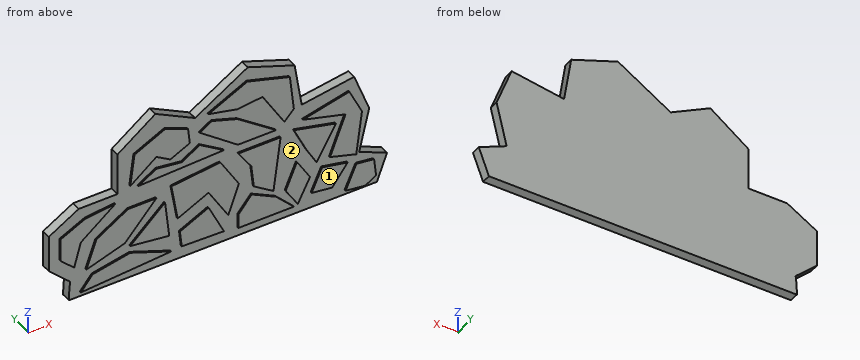
from build123d import *

# Parameters (mm, degrees)
F1_DEPTH = 3
F3_DEPTH = 0.5


with BuildPart() as f1:
    # F0 (on Front) → F1 (new body)
    with BuildSketch(Plane.XZ):
        with BuildLine():
            ThreePointArc((-49.601689, 6.298609), (-49.900323, 3.155595), (-50, 0))
            Line((-50, 0), (50, 0))
            Line((50, 0), (53.269234, 8.75))
            Line((53.269234, 8.75), (44.23077, 12.788462))
            Line((44.23077, 12.788462), (47.500003, 26.634617))
            Line((47.500003, 26.634617), (42.601875, 39.515073))
            Line((42.601875, 39.515073), (25.576925, 36.826923))
            Line((25.576925, 36.826923), (23.269232, 51.44231))
            Line((23.269232, 51.44231), (8.076922, 57.019234))
            Line((8.076922, 57.019234), (-9.038462, 46.442311))
            Line((-9.038462, 46.442311), (-21.923078, 53.17308))
            Line((-21.923078, 53.17308), (-34.230769, 44.134621))
            Line((-34.230769, 44.134621), (-34.230769, 30.420949))
            Line((-34.230769, 30.420949), (-46.853391, 30.420949))
            Line((-46.853391, 30.420949), (-56.538463, 24.71154))
            Line((-56.538463, 24.71154), (-56.538463, 12.788462))
            Line((-56.538463, 12.788462), (-49.601689, 6.298609))
        make_face()
    extrude(amount=F1_DEPTH)

    # F2 (on face) → F3 (join)
    with BuildSketch(Plane.XZ.offset(3)):
        Polygon((-53.070076, 15.257269), (-48.621472, 11.095279), (-46.445761, 18.982239), (-35.295229, 27.685093), (-44.949956, 26.597237), (-53.070076, 22.653757), align=None)
        Polygon((-29.040052, 42.235177), (-30.399874, 31.900536), (-21.923078, 38.563661), (-17.39964, 35.819323), (-11.0592, 38.898515), (-11.634346, 44.002943), (-19.030639, 47.09618), align=None)
        Polygon((7.616132, 52.555275), (-4.971225, 46.442311), (4.379547, 44.303863), (12.570463, 45.226783), (19.641532, 33.668306), (22.715791, 36.895224), (21.409299, 48.490353), align=None)
        Polygon((40.718757, 35.436071), (25.624743, 31.900536), (39.494917, 28.09304), (34.463577, 15.310723), (42.973845, 12.788462), (44.837793, 26.95446), align=None)
        Polygon((48.750002, 8.710921), (43.030452, 9.463494), (39.500919, 1.540576), (45.901778, 0.698357), (49.410935, 2.845136), align=None)
        Polygon((35.143491, 4.432157), (40.174823, 11.095279), (31.879921, 12.788462), (28.481199, 5.308775), align=None)
        Polygon((26.872491, 20.893696), (30.112153, 15.310723), (36.367327, 26.18929), (22.715791, 29.45286), align=None)
        Polygon((4.547521, 31.900536), (16.921889, 31.900536), (4.411539, 40.875357), (-3.883368, 43.594997), (-7.848335, 41.16937), align=None)
        Polygon((-27.739104, 30.859229), (0, 31.900536), (-7.826848, 36.895224), (-13.655543, 33.329433), (-21.923078, 34.417268), align=None)
        Polygon((-41.414421, 17.894384), (-44.677991, 8.75), (-32.16764, 12.788462), (-21.923078, 24.215545), (-31.081754, 24.215545), align=None)
        Polygon((-1.151366, 28.119329), (-17.073629, 26.325272), (-15.014787, 14.319498), (-4.971225, 19.197085), (1.419934, 8.75), (4.85837, 18.295721), align=None)
        Polygon((-19.11336, 21.565899), (-30.399874, 11.095279), (-17.74971, 9.463494), align=None)
        Polygon((18.417694, 28.77295), (4.683502, 28.77295), (8.887457, 22.653757), (9.71484, 15.310723), (16.091682, 11.095279), align=None)
        Polygon((23.720995, 18.030366), (20.049477, 9.463494), (23.992959, 3.3443), (27.963636, 11.095279), align=None)
        Polygon((9.034931, 12.788462), (4.683502, 7.559745), (4.683502, 2.936354), (22.715791, 2.936354), (16.921889, 8.75), align=None)
        Polygon((-13.684647, 4.099629), (0, 3.752247), (-4.971225, 13.98862), (-14.289026, 9.463494), align=None)
        Polygon((-46.445761, 1.576533), (-17.073629, 3.752247), (-30.399874, 8.75), (-42.638261, 6.298609), align=None)
    extrude(amount=F3_DEPTH)


solid = f1.part
Part model, mm, in its own coordinate system. Face numbers are marked on the shaded views. Coordinates: 2 decimals unless noted, no trailing zeros. Loops run counter-clockwise (first coordinate to the right, second up) from the corner with the lowest first, then second, coordinate; pieces in that order, holes last. Notation, with made-up numbers: M 52.5,-4 L 62.5,-4 A21 cw 62.5,31 Z; hole C 8.5,77 d2. An arc over 180 degrees is marked long. Use a Markdown table: item, result. Add a question column.
Q1. Probe L1, parallel to Z at x = -10, y = -3.3; L2, parallel to Y at x = -22.5, z = 45.5; L3, parallel to Z at x = -39.5, y = -0.4. List the from-to ranges inside material, lowest first.
Q2. Cut at A-A (y = -1.25). Write the cut outline in (x, z), and give its area (3 significant figures).
Q3. Cut at B-B (x = 14). Write the cut outline in (y, z), and give its area (3 significant figures).
Q4. Pin check, flat tips, straight feed: P1, Ø1, axis at y = -2.5, z = 43, coming from the -X side; P2, Ø3, axis at x = -21, z = 48, coming from the -Y side; P3, Ø0.6, axis at x = -25.5, y = -3, coming from the +Z side; P4, Ø3, axis at x = -32.5, z = 23, coming from the +Y side. Stop position of each tip, or through.
Q5. Mould opens along X. For the marked faces 1 and 2 say: +X half, -X half, draft (parallel to the pull), parting line (faces both ways), or undercut.
Worked out:
| question | item | result |
|---|---|---|
| 1 | L1 | z = 4.01 to 11.55, 16.75 to 27.12, 31.53 to 35.57 |
| 1 | L2 | y = -3 to 0 |
| 1 | L3 | z = 0 to 30.42 |
| 2 | outline | M -56.54,12.79 L -49.6,6.3 A50 ccw -50,0 L 50,0 L 53.27,8.75 L 44.23,12.79 L 47.5,26.63 L 42.6,39.52 L 25.58,36.83 L 23.27,51.44 L 8.08,57.02 L -9.04,46.44 L -21.92,53.17 L -34.23,44.13 L -34.23,30.42 L -46.85,30.42 L -56.54,24.71 Z |
| 2 | area | 4,470 mm2 |
| 3 | outline | M -3.5,2.94 L -3,2.94 L -3,0 L 0,0 L 0,54.84 L -3,54.84 L -3,50.67 L -3.5,50.67 L -3.5,42.89 L -3,42.89 L -3,34 L -3.5,34 L -3.5,31.9 L -3,31.9 L -3,28.77 L -3.5,28.77 L -3.5,12.48 L -3,12.48 L -3,10.25 L -3.5,10.25 Z |
| 3 | area | 181 mm2 |
| 4 | P1 | stops at x = -34.23 |
| 4 | P2 | stops at y = -3 |
| 4 | P3 | stops at z = 50.77 |
| 4 | P4 | stops at y = 0 |
| 5 | face 1 | draft |
| 5 | face 2 | undercut |
